Check sheet for the modelled part. Datum: model origin and axes. Units: mm. A direction names the side the tool comes from. Give positions to 0.01 mm unless a question says otherwise; leave off trailing zeros. Write each loop counter-clockwise with the first axis right and the second up, starting at its lowest first coordinate (ties: lowest second). Pieces come first, ordered by that corner, then holes. Notation, with made-up numbers: M 70,-25.75 L 81,-25.75 A12 cw 81,-20.75 Z; hole C 0,13.5 d1. An arc over 180 degrees is marked long. Write item = value, one per line. Start each with the question number.
1) Mould release check, pull along X, two halves, no side actions. Record for faces 1 (the flat face through (-10, -4, 0)), 2 (the flat face through (25, 1, 0)), 3 (the flat face through (17, -22.2, 0)), 4 (the flat face through (-25, 2, 0)): released by +X, released by -X, zero draft, split by the parting line, or undercut.
2) Scan lines: line 1 along X through (y, z) = (-2.5, -6.75); line 2 along Y through (x, z) = (-5, 7); line 3 along X through (y, z) = (-8.5, -0.75). Record each from-to range of solid material in increasing order. Write a range as [from, to].
3) Access from +Z, -Z, +X, -X, +Y, -Y to the whole of each face (thin tool, end or side, straight path). Record for faces 5 (the cylindrical face through (13.04, -14.1, -0.59)), 6 (the flat face through (0, 2, -8.5)), 7 (the flat face through (10, -4, 0)).
4) Cross-section at D-D, the plane z = -6. Record the cut outline in (x, y).
5) Cross-section at B-B, the plane z = 0. Record the cut outline in (x, y).
6) Cross-section at C-C, the plane x = -17.5. Record the cut outline in (y, z), plus the area to 3 significant figures.
7) Go/stop test with flat-tipped pins: pin 1 (1 mm diameter, centred on y = -10.5, z = 4, fed in from -X); pin 2 (4 mm diameter, centred on y = -12, z = -6, fed in from +X); pin 3 (5 mm diameter, centred on x = -2, z = -2, fed in from -Y). Record where each tip stops, or that it passes through.
8) Cross-section at A-A, the plane y = -9. Record the cut outline in (x, z).
```python
from build123d import *

# Parameters (mm, degrees)
SKETCH1_W           = 50
SKETCH1_H           = 17
BOSS_EXTRUDE1_DEPTH = 10
SKETCH2_W           = 15
SKETCH2_H           = 17
BOSS_EXTRUDE2_DEPTH = 7.2
SKETCH3_R           = 4.5
BOSS_EXTRUDE3_DEPTH = 15
FILLET1_R           = 1


with BuildPart() as part:
    # Sketch1 → Boss-Extrude1 (new body)
    with BuildSketch(Plane(origin=(0, 0, 0), x_dir=(1, 0, 0), z_dir=(0, 1, 0))):
        Rectangle(SKETCH1_W, SKETCH1_H)
    extrude(amount=BOSS_EXTRUDE1_DEPTH)

    # Sketch2 → Boss-Extrude2 (add)
    with BuildSketch(Plane.XZ):
        with Locations((-17.5, 0)):
            Rectangle(SKETCH2_W, SKETCH2_H)
        with Locations((17.5, 0)):
            Rectangle(SKETCH2_W, SKETCH2_H)
    extrude(amount=BOSS_EXTRUDE2_DEPTH)

    # Sketch3 → Boss-Extrude3 (add)
    with BuildSketch(Plane.XZ.offset(7.2)):
        with Locations(Location((-17.5, 0, 0), (0, 0, 90))):
            Circle(SKETCH3_R)
        with Locations(Location((17.5, 0, 0), (0, 0, 90))):
            Circle(SKETCH3_R)
    extrude(amount=BOSS_EXTRUDE3_DEPTH)

    # Fillet1
    fillet1_edges = [part.edges().sort_by_distance(p)[0] for p in [
        (-17.5, -22.2, -4.5),
        (17.5, -22.2, -4.5),
    ]]
    fillet(fillet1_edges, radius=FILLET1_R)


solid = part.part
```
Reply:
q1.face_1 = undercut
q1.face_2 = released by +X
q1.face_3 = zero draft
q1.face_4 = released by -X
q2.line_1 = [-25, -10], [10, 25]
q2.line_2 = [0, 10]
q2.line_3 = [-21.94, -13.06], [13.06, 21.94]
q3.face_5 = -Y
q3.face_6 = -Z, +X, -X, +Y, -Y
q3.face_7 = +Z, -Z, -Y
q4.outline = M -25,-7.2 L -10,-7.2 L -10,0 L 10,0 L 10,-7.2 L 25,-7.2 L 25,10 L -25,10 Z
q5.outline = M -25,-7.2 L -22,-7.2 L -22,-21.2 A1 ccw -21,-22.2 L -14,-22.2 A1 ccw -13,-21.2 L -13,-7.2 L -10,-7.2 L -10,0 L 10,0 L 10,-7.2 L 13,-7.2 L 13,-21.2 A1 ccw 14,-22.2 L 21,-22.2 A1 ccw 22,-21.2 L 22,-7.2 L 25,-7.2 L 25,10 L -25,10 Z
q6.outline = M -22.2,-3.5 A1 ccw -21.2,-4.5 L -7.2,-4.5 L -7.2,-8.5 L 10,-8.5 L 10,8.5 L -7.2,8.5 L -7.2,4.5 L -21.2,4.5 A1 ccw -22.2,3.5 Z
q6.area = 427 mm2
q7.pin_1 = -20.33
q7.pin_2 = 19.56
q7.pin_3 = 0
q8.outline = C -17.5,0 d9; C 17.5,0 d9
